Read the model definition and answer for the solid it produces. Units are mm, in the model's axes. Coordinates: 2 decimals unless noted, no trailing zeros. Loops run counter-clockwise (first coordinate to the right, second up) from the corner with the lowest first, then second, coordinate; pieces in that order, holes last.
Q1. Section C-C (y = -39.5) is taken. Give the vertices of the cut face in (x, z).
Q2. The mould has two halves that part along Z. Classify faces 1 (the face through (-59, 0, -98)), 2 (the face through (95.38, -24.65, 30.04)), 3 (the face through (188.375, -24.65, 99.3)), 4 (the face through (-3, -25, -150)): pulls with the +Z half, pulls with the -Z half, needs draft (parallel to the pull), parting line crosses it, or undercut.
Q3. Section A-A (x = 175) is taken. Give the vertices of the cut face in (y, z), then the cut area to 3 significant figures.
Q4. Straight lines are drawn through the part: line 1 (Z direction, x = 0, y = -37); line 2 (Z direction, x = -182.5, y = -27); line 3 (X direction, y = -45, z = -68). For each, find the intervals that lie inside material, in ascending order.
Q5. Flat-ended cylindrical pins translate along their axes: P1, Ø12, axis at x = 133.5, y = -22.5, coming from the +Z side; P2, Ø1.5, axis at x = -160, y = -31.5, coming from the +Z side; P3, Ø1.5, axis at y = -41, z = 85.5, coming from the -X side. Find the tip coordinate at first contact, or state that the pin passes through.
Q6. Section D-D (z = -50) is taken. Give the vertices of the cut face in (x, y).
Q7. Section B-B (z = 0) is taken. Give the vertices of the cut face in (x, y).
from build123d import *

# Parameters (mm, degrees)
F0_R     = 37.5
F0_R_2   = 100
F1_DEPTH = 50


with BuildPart() as f1:
    # F0 (on Front) → F1 (new body)
    with BuildSketch(Plane.XZ):
        Polygon((250, 50), (125, 150), (-125, 150), (-250, 50), (-250, 0), (-250, -150), (0, -150), (175, -150), (250, -150), (250, -50), align=None)
        with Locations((-175, -50)):
            Circle(F0_R, mode=Mode.SUBTRACT)
        with Locations((175, -50)):
            Circle(F0_R, mode=Mode.SUBTRACT)
        Circle(F0_R_2, mode=Mode.SUBTRACT)
    extrude(amount=F1_DEPTH)


solid = f1.part
Numbers:
1. outline: (-250, -150) - (250, -150) - (250, 50) - (125, 150) - (-125, 150) - (-250, 50) - close; hole circle Ø75 at (-175, -50); hole circle Ø200 at (0, 0); hole circle Ø75 at (175, -50)
2. face 1: needs draft
2. face 2: undercut
2. face 3: pulls with the +Z half
2. face 4: pulls with the -Z half
3. outline: (-50, -150) - (0, -150) - (0, -87.5) - (-50, -87.5) - close; (-50, -12.5) - (0, -12.5) - (0, 110) - (-50, 110) - close
3. area: 9,250 mm2
4. line 1: z = -150 to -100, 100 to 150
4. line 2: z = -150 to -86.74, -13.26 to 104
4. line 3: x = -250 to -207.9, -142.1 to -73.32, 73.32 to 142.1, 207.9 to 250
5. P1: stops at z = 148
5. P2: stops at z = 122.6
5. P3: stops at x = -206.56
6. outline: (-250, -50) - (-212.5, -50) - (-212.5, 0) - (-250, 0) - close; (-137.5, -50) - (-86.6, -50) - (-86.6, 0) - (-137.5, 0) - close; (86.6, -50) - (137.5, -50) - (137.5, 0) - (86.6, 0) - close; (212.5, -50) - (250, -50) - (250, 0) - (212.5, 0) - close
7. outline: (-250, -50) - (-100, -50) - (-100, 0) - (-250, 0) - close; (100, -50) - (250, -50) - (250, 0) - (100, 0) - close
